Geometry: final body of the model. Coordinates: model frame, mm. Face numbers are marked on the shaded views. Give positions to 0.01 mm unless a question says otherwise; leave off trailing zeros. One line per question, with ' | ' between items. Start each with the question number.
Item 1: Pin query (flat end, axial travel): P1, Ø1, axis at y = -7.5, z = 3, coming from the +X side; P2, Ø3, axis at y = -8, z = 1.5, coming from the +X side; P3, Ø1, axis at x = -7, z = 4.5, coming from the +Y side. Return the tip coordinate at first contact, or that it passes through.
Item 2: Material intervals for line 1 along X through (y, z) = (-12, 2.25); line 2 along Y through (x, z) = (0, 2.55); line 3 along X through (y, z) = (11.5, 4.75), sorted ascending. Write a range as [from, to].
Item 3: Mould query, pull axis X, two halves, no side actions, for the marked faces 1 and 2. Classes: released by +X, released by -X, zero draft, split by the parting line, or undercut.
from build123d import *

# Parameters (mm, degrees)
SKETCH1_R           = 4
BOSS_EXTRUDE1_DEPTH = 5


with BuildPart() as part:
    # Sketch1 → Boss-Extrude1 (new body)
    with BuildSketch(Plane.XY):
        with BuildLine():
            add(Edge.make_bspline(
                [(0, 15), (2.939188217, 14.272515919), (1.529993599, 11.135281605), (3.13745877, 9.656105206)],
                knots=[0, 0, 0, 0, 0.926158454, 0.926158454, 0.926158454, 0.926158454], degree=3))
            add(Edge.make_bspline(
                [(0, 15), (-2.939188224, 14.272515918), (-1.529993593, 11.13528159), (-3.137458782, 9.656105196)],
                knots=[0, 0, 0, 0, 0.926158457, 0.926158457, 0.926158457, 0.926158457], degree=3))
            add(Edge.make_bspline(
                [(-8.816778784, 12.135254916), (-6.01132116, 13.274319416), (-5.307363487, 9.907939744), (-3.137458785, 9.656105208)],
                knots=[0, 0, 0, 0, 0.926158452, 0.926158452, 0.926158452, 0.926158452], degree=3))
            add(Edge.make_bspline(
                [(-8.816778784, 12.135254916), (-10.767027588, 9.819096444), (-7.782945131, 8.109324382), (-8.213973699, 5.967801216)],
                knots=[0, 0, 0, 0, 0.926158454, 0.926158454, 0.926158454, 0.926158454], degree=3))
            add(Edge.make_bspline(
                [(-14.265847744, 4.635254916), (-12.66571016, 7.205784078), (-10.117488108, 4.896101636), (-8.213973699, 5.967801216)],
                knots=[0, 0, 0, 0, 0.926158454, 0.926158454, 0.926158454, 0.926158454], degree=3))
            add(Edge.make_bspline(
                [(-14.265847744, 4.635254916), (-14.482228378, 1.615115865), (-11.063076155, 1.98588087), (-10.153029858, 0)],
                knots=[0, 0, 0, 0, 0.926158454, 0.926158454, 0.926158454, 0.926158454], degree=3))
            add(Edge.make_bspline(
                [(-14.265847744, -4.635254916), (-14.482228378, -1.615115865), (-11.063076155, -1.98588087), (-10.153029858, 0)],
                knots=[0, 0, 0, 0, 0.926158454, 0.926158454, 0.926158454, 0.926158454], degree=3))
            add(Edge.make_bspline(
                [(-14.265847744, -4.635254916), (-12.665710158, -7.205784082), (-10.117488099, -4.896101628), (-8.21397369, -5.967801222)],
                knots=[0, 0, 0, 0, 0.926158456, 0.926158456, 0.926158456, 0.926158456], degree=3))
            add(Edge.make_bspline(
                [(-8.816778784, -12.135254916), (-10.767027584, -9.819096448), (-7.782945142, -8.109324388), (-8.213973697, -5.967801228)],
                knots=[0, 0, 0, 0, 0.926158453, 0.926158453, 0.926158453, 0.926158453], degree=3))
            add(Edge.make_bspline(
                [(-8.816778784, -12.135254916), (-6.01132116, -13.274319416), (-5.307363487, -9.907939744), (-3.137458785, -9.656105208)],
                knots=[0, 0, 0, 0, 0.926158452, 0.926158452, 0.926158452, 0.926158452], degree=3))
            add(Edge.make_bspline(
                [(0, -15), (-2.939188224, -14.272515918), (-1.529993593, -11.13528159), (-3.137458782, -9.656105196)],
                knots=[0, 0, 0, 0, 0.926158457, 0.926158457, 0.926158457, 0.926158457], degree=3))
            add(Edge.make_bspline(
                [(0, -15), (2.939188224, -14.272515918), (1.529993593, -11.13528159), (3.137458782, -9.656105196)],
                knots=[0, 0, 0, 0, 0.926158457, 0.926158457, 0.926158457, 0.926158457], degree=3))
            add(Edge.make_bspline(
                [(8.816778784, -12.135254916), (6.01132116, -13.274319416), (5.307363487, -9.907939744), (3.137458785, -9.656105208)],
                knots=[0, 0, 0, 0, 0.926158452, 0.926158452, 0.926158452, 0.926158452], degree=3))
            add(Edge.make_bspline(
                [(8.816778784, -12.135254916), (10.767027588, -9.819096444), (7.782945131, -8.109324382), (8.213973699, -5.967801216)],
                knots=[0, 0, 0, 0, 0.926158454, 0.926158454, 0.926158454, 0.926158454], degree=3))
            add(Edge.make_bspline(
                [(14.265847744, -4.635254916), (12.66571016, -7.205784078), (10.117488108, -4.896101636), (8.213973699, -5.967801216)],
                knots=[0, 0, 0, 0, 0.926158454, 0.926158454, 0.926158454, 0.926158454], degree=3))
            add(Edge.make_bspline(
                [(14.265847744, -4.635254916), (14.482228378, -1.615115865), (11.063076155, -1.98588087), (10.153029858, 0)],
                knots=[0, 0, 0, 0, 0.926158454, 0.926158454, 0.926158454, 0.926158454], degree=3))
            add(Edge.make_bspline(
                [(14.265847744, 4.635254916), (14.482228378, 1.615115865), (11.063076155, 1.98588087), (10.153029858, 0)],
                knots=[0, 0, 0, 0, 0.926158454, 0.926158454, 0.926158454, 0.926158454], degree=3))
            add(Edge.make_bspline(
                [(14.265847744, 4.635254916), (12.665710158, 7.205784082), (10.117488099, 4.896101628), (8.21397369, 5.967801222)],
                knots=[0, 0, 0, 0, 0.926158456, 0.926158456, 0.926158456, 0.926158456], degree=3))
            add(Edge.make_bspline(
                [(8.816778784, 12.135254916), (10.767027584, 9.819096448), (7.782945142, 8.109324388), (8.213973697, 5.967801228)],
                knots=[0, 0, 0, 0, 0.926158453, 0.926158453, 0.926158453, 0.926158453], degree=3))
            add(Edge.make_bspline(
                [(8.816778784, 12.135254916), (6.011321153, 13.274319419), (5.307363484, 9.907939729), (3.13745877, 9.656105206)],
                knots=[0, 0, 0, 0, 0.926158454, 0.926158454, 0.926158454, 0.926158454], degree=3))
        make_face()
        Circle(SKETCH1_R, mode=Mode.SUBTRACT)
    extrude(amount=BOSS_EXTRUDE1_DEPTH)


solid = part.part
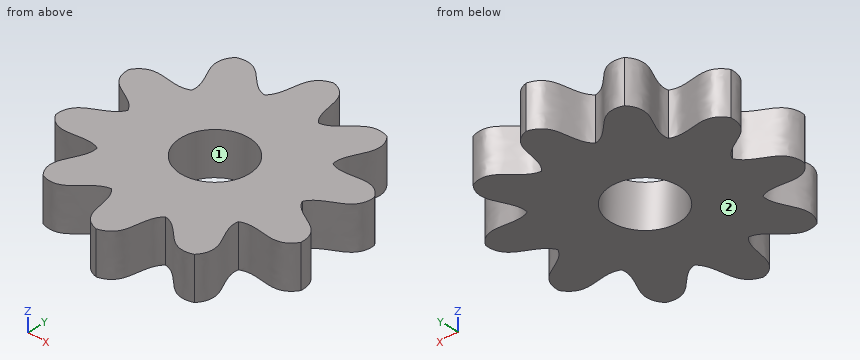
Result sheet:
1) P1: stops at x = 8.61 | P2: stops at x = 9.3 | P3: stops at y = 12.36
2) line 1: x = [-8.93, -6.49], [-2.18, 2.18], [6.49, 8.93] | line 2: y = [-15, -4], [4, 15] | line 3: x = [-9.24, -5.83], [-2.27, 2.27], [5.83, 9.24]
3) face 1: undercut | face 2: zero draft
